from build123d import *

# Parameters (mm, degrees)
SKETCH_1_R      = 2.65
SKETCH_1_R_2    = 1.5
EXTRUDE_1_DEPTH = 156


with BuildPart() as part:
    # 草图1 → 凸台-拉伸1 (new, symmetric)
    with BuildSketch(Plane.XY):
        with BuildLine():
            Line((3.142893219, 3.85), (-3.142893219, 3.85))
            Line((-3.142893219, 3.85), (-5.5, 6.207106781))
            Line((-5.5, 6.207106781), (-5.5, 8.3))
            Line((-5.5, 8.3), (-3.1, 8.3))
            Line((-3.1, 8.3), (-3.1, 9.5))
            Line((-3.1, 9.5), (-3.6, 9.5))
            Line((-3.6, 9.5), (-3.6, 9.7))
            ThreePointArc((-3.6, 9.7), (-3.687867966, 9.912132034), (-3.9, 10))
            Line((-3.9, 10), (-8.5, 10))
            ThreePointArc((-8.5, 10), (-9.560660172, 9.560660172), (-10, 8.5))
            Line((-10, 8.5), (-10, 3.9))
            ThreePointArc((-10, 3.9), (-9.912132034, 3.687867966), (-9.7, 3.6))
            Line((-9.7, 3.6), (-9.5, 3.6))
            Line((-9.5, 3.6), (-9.5, 3.1))
            Line((-9.5, 3.1), (-8.3, 3.1))
            Line((-8.3, 3.1), (-8.3, 5.5))
            Line((-8.3, 5.5), (-6.207106781, 5.5))
            Line((-6.207106781, 5.5), (-3.85, 3.142893219))
            Line((-3.85, 3.142893219), (-3.85, -3.142893219))
            Line((-3.85, -3.142893219), (-6.207106781, -5.5))
            Line((-6.207106781, -5.5), (-8.3, -5.5))
            Line((-8.3, -5.5), (-8.3, -3.1))
            Line((-8.3, -3.1), (-9.5, -3.1))
            Line((-9.5, -3.1), (-9.5, -3.6))
            Line((-9.5, -3.6), (-9.7, -3.6))
            ThreePointArc((-9.7, -3.6), (-9.912132034, -3.687867966), (-10, -3.9))
            Line((-10, -3.9), (-10, -8.5))
            ThreePointArc((-10, -8.5), (-9.560660172, -9.560660172), (-8.5, -10))
            Line((-8.5, -10), (-3.9, -10))
            ThreePointArc((-3.9, -10), (-3.687867966, -9.912132034), (-3.6, -9.7))
            Line((-3.6, -9.7), (-3.6, -9.5))
            Line((-3.6, -9.5), (-3.1, -9.5))
            Line((-3.1, -9.5), (-3.1, -8.3))
            Line((-3.1, -8.3), (-5.5, -8.3))
            Line((-5.5, -8.3), (-5.5, -6.207106781))
            Line((-5.5, -6.207106781), (-3.142893219, -3.85))
            Line((-3.142893219, -3.85), (3.142893219, -3.85))
            Line((3.142893219, -3.85), (5.5, -6.207106781))
            Line((5.5, -6.207106781), (5.5, -8.3))
            Line((5.5, -8.3), (3.1, -8.3))
            Line((3.1, -8.3), (3.1, -9.5))
            Line((3.1, -9.5), (3.6, -9.5))
            Line((3.6, -9.5), (3.6, -9.7))
            ThreePointArc((3.6, -9.7), (3.687867966, -9.912132034), (3.9, -10))
            Line((3.9, -10), (8.5, -10))
            ThreePointArc((8.5, -10), (9.560660172, -9.560660172), (10, -8.5))
            Line((10, -8.5), (10, -3.9))
            ThreePointArc((10, -3.9), (9.912132034, -3.687867966), (9.7, -3.6))
            Line((9.7, -3.6), (9.5, -3.6))
            Line((9.5, -3.6), (9.5, -3.1))
            Line((9.5, -3.1), (8.3, -3.1))
            Line((8.3, -3.1), (8.3, -5.5))
            Line((8.3, -5.5), (6.207106781, -5.5))
            Line((6.207106781, -5.5), (3.85, -3.142893219))
            Line((3.85, -3.142893219), (3.85, 3.142893219))
            Line((3.85, 3.142893219), (6.207106781, 5.5))
            Line((6.207106781, 5.5), (8.3, 5.5))
            Line((8.3, 5.5), (8.3, 3.1))
            Line((8.3, 3.1), (9.5, 3.1))
            Line((9.5, 3.1), (9.5, 3.6))
            Line((9.5, 3.6), (9.7, 3.6))
            ThreePointArc((9.7, 3.6), (9.912132034, 3.687867966), (10, 3.9))
            Line((10, 3.9), (10, 8.5))
            ThreePointArc((10, 8.5), (9.560660172, 9.560660172), (8.5, 10))
            Line((8.5, 10), (3.9, 10))
            ThreePointArc((3.9, 10), (3.687867966, 9.912132034), (3.6, 9.7))
            Line((3.6, 9.7), (3.6, 9.5))
            Line((3.6, 9.5), (3.1, 9.5))
            Line((3.1, 9.5), (3.1, 8.3))
            Line((3.1, 8.3), (5.5, 8.3))
            Line((5.5, 8.3), (5.5, 6.207106781))
            Line((5.5, 6.207106781), (3.142893219, 3.85))
        make_face()
        Circle(SKETCH_1_R, mode=Mode.SUBTRACT)
        with Locations((-7.75, 7.75)):
            Circle(SKETCH_1_R_2, mode=Mode.SUBTRACT)
        with Locations((7.75, 7.75)):
            Circle(SKETCH_1_R_2, mode=Mode.SUBTRACT)
        with Locations((7.75, -7.75)):
            Circle(SKETCH_1_R_2, mode=Mode.SUBTRACT)
        with Locations((-7.75, -7.75)):
            Circle(SKETCH_1_R_2, mode=Mode.SUBTRACT)
    extrude(amount=EXTRUDE_1_DEPTH, both=True)


solid = part.part
Read the model definition and answer for the solid it produces. Units are mm, in the model's axes. A direction names the side the tool comes from. Round coordinates to 2 decimals unless told otherwise and drop trailing zeros. Write each loop counter-clockwise with the first axis right and the second up, starting at its lowest first coordinate (ties: lowest second). Pieces come first, ordered by that corner, then holes.
1. Given pin 1 Ø2.5 at (x, y) = (-7.75, 7.75) entering from +Z; pin 2 Ø3 at (x, z) = (-1.5, 37) entering from +Y; pin 3 Ø4 at (x, z) = (1.5, -47) entering from -Y; pin 4 Ø0.6 at (y, z) = (-3.5, -53) entering from -X, each flat-ended and moving along its own axis, determine where each tip first touches the part or whether it passes through.
2. Determine the mould class of faces 1 (the face through (-2, 2, 156)), 2 (the face through (-3.85, 0, 2)), 3 (the face through (0, -3.85, 2)), 4 (the face through (2.45, -1.01, -2.18)) for opening direction Y: pulls with the +Y half, pulls with the -Y half, needs draft (parallel to the pull), parting line crosses it, or undercut.
3. The part is cut by section C-C, the plane z = 119. State how many separate pieces and enclosed holes the cut face has, then the cut area to 3 significant figures.
4. The part is cut by section A-A, the plane x = 0. Determine the outline of the cut face in (y, z).
5. Straight lines are drawn through the part: L1, parallel to X at y = -8, z = 26.5; L2, parallel to Y at x = 0, z = 76. For each, find the intervals that lie inside material, in ascending order.
6. Which of the six approach directions +Z, -Z, +X, -X, +Y, -Y give full straight-line access (tool end or side, diameter ignored) to faces 5 (the face through (3.85, 0, 2)), 6 (the face through (-2, 2, -156)), 7 (the face through (0, 3.85, 2))?
Values:
1. pin 1: passes through
1. pin 2: stops at y = 3.85
1. pin 3: stops at y = -9.5
1. pin 4: stops at x = -9.98
2. face 1: needs draft
2. face 2: undercut
2. face 3: pulls with the -Y half
2. face 4: undercut
3. separate pieces: 1
3. enclosed holes: 5
3. area: 130 mm2
4. outline: (-3.85, -156) - (-2.65, -156) - (-2.65, 156) - (-3.85, 156) - close; (2.65, -156) - (3.85, -156) - (3.85, 156) - (2.65, 156) - close
5. L1: x = -10 to -9.23, -6.27 to -5.5, 5.5 to 6.27, 9.23 to 10
5. L2: y = -3.85 to -2.65, 2.65 to 3.85
6. face 5: +Z, -Z, +X
6. face 6: -Z, +X, -X, +Y, -Y
6. face 7: +Z, -Z, +Y
